Source: CAD feature listing. Evaluate the final solid. Frame: model axes, mm. Face numbers are marked on the shaded views. Give positions to 0.01 mm unless a question says otherwise; leave off trailing zeros. Order: outer loops, then holes, each group sorted by start corner. A loop starts at its lowest first (then second) coordinate and runs counter-clockwise, first axis right, second up. Notation, with made-up numbers: (68, 24) - (108, 24) arc R25 ccw to (108, 45) - close; hole circle Ø2 at (84, -21). An arc over 180 degrees is marked (long way). Write each question's results on one line, items separated by ' | '. Start each with the question number.
Item 1: Section A-A on z = -6.5. Output: boundary loops of the cut face in (x, y).
Item 2: Section B-B on y = 11.5. Output: boundary loops of the cut face in (x, z), and give its area (3 significant figures).
Item 3: Mould query, pull axis X, two halves, no side actions, for the marked faces 1, 2 and 3. Classes: released by +X, released by -X, zero draft, split by the parting line, or undercut.
Item 4: Line query: line 1 along X through (y, z) = (54.5, -15); line 2 along Z through (x, y) = (287, 40). Output: solid intervals per line, ascending.
Item 5: Contact query for a flat-ended pin moving along its axis: pin 1 Ø17.5 at (x, y) = (379.5, 26) entering from +Z. Output: stop coordinate, or through.
Item 6: Section C-C on x = 376. Output: boundary loops of the cut face in (y, z).
Autodesk Inventor part; units mm, degrees
ref_plane "YZ Plane" through (0, 0, 0) normal (1, 0, 0) x (0, 1, 0)
ref_plane "XZ Plane" through (0, 0, 0) normal (0, 1, 0) x (-1, 0, 0)
ref_plane "XY Plane" through (0, 0, 0) normal (0, 0, 1) x (1, 0, 0)
sketch "Sketch1" plane through (0, 0, 0) normal (0, 1, 0) x (-1, 0, 0)
  line L0 (0, 0) -> (-690, 0)
  line L1 (-690, 0) -> (-690, -40)
  line L2 (-690, -40) -> (0, -40)
  line L3 (0, -40) -> (0, 0)
  dimension "d0" = 690
  dimension "d1" = 40
extrude "Extrusion1" add sketch "Sketch1" along normal blind 60
sketch "Sketch3" plane through (0, 60, 0) normal (0, 1, 0) x (1, 0, 0)
  circle A0 centre (380.6828, 16.7692) radius 7.5
  line L0 (368.0221, 25.8207) -> (368.0221, 1.9407)
  line L1 (393.2421, 25.8207) -> (368.0221, 25.8207)
  line L2 (393.2421, 1.9407) -> (393.2421, 25.8207)
  line L3 (368.0221, 1.9407) -> (393.2421, 1.9407)
  line L4 (0, 0) -> (690, 0)
  line L5 (690, 40) -> (0, 40)
  line L6 (0, 40) -> (0, 0)
  line L7 (368.0221, 1.9407) -> (363.0221, 1.9407)
  line L8 (368.0221, 25.8207) -> (368.0221, 30.8207)
  line L9 (393.2421, 1.9407) -> (398.2421, 1.9407)
  line L10 (363.0221, 1.9407) -> (363.0221, 0)
  line L11 (398.2421, 1.9407) -> (398.2421, 0)
  line L12 (363.0221, 0) -> (398.2421, 0)
  line L13 (398.2421, 0) -> (398.2421, 30.8207)
  line L14 (398.2421, 30.8207) -> (363.0221, 30.8207)
  line L15 (363.0221, 30.8207) -> (363.0221, 0)
  point P0 (0, 40)
  dimension "d6" = 5
  dimension "d7" = 5
  dimension "d8" = 5
extrude "Extrusion3" cut sketch "Sketch3" against normal blind 60 contours A0 | L1 L2 L3 L0 | L8 L14 L13 L9 L2 L1 | L0 L7 L15 L14 L8 | L3 L9 L11 L4 L10 L7
sketch "Sketch4" plane through (0, 0, 0) normal (0, -1, 0) x (1, 0, 0)
  line L0 (0, 0) -> (363.0221, 0)
  line L1 (333.0221, 0) -> (268.0221, 0)
  line L2 (268.0221, 0) -> (268.0221, -25)
  line L3 (268.0221, -25) -> (333.0221, -25)
  line L4 (333.0221, -25) -> (333.0221, 0)
  line L5 (363.0221, -30.8207) -> (363.0221, 0)
  dimension "d11" = 65
  dimension "d12" = 25
  dimension "d13" = 30
extrude "Extrusion4" cut sketch "Sketch4" against normal blind 60
properties part number "Cadru_4"
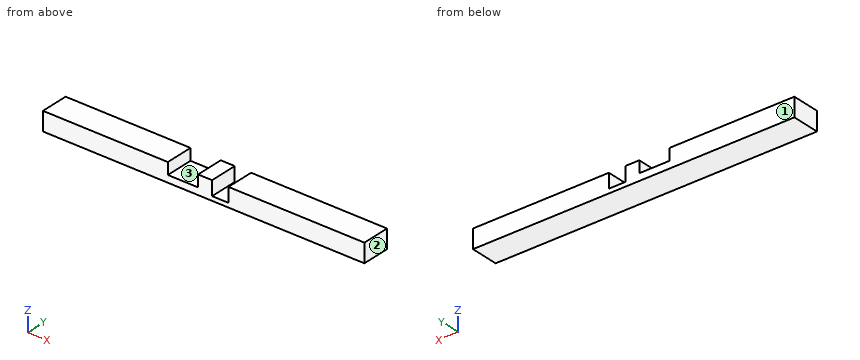
Evaluation:
1) outline: (0, 0) - (268.02, 0) - (268.02, 60) - (0, 60) - close; (333.02, 0) - (363.02, 0) - (363.02, 60) - (333.02, 60) - close; (398.24, 0) - (690, 0) - (690, 60) - (398.24, 60) - close
2) outline: (0, -40) - (690, -40) - (690, 0) - (398.24, 0) - (398.24, -30.82) - (363.02, -30.82) - (363.02, 0) - (333.02, 0) - (333.02, -25) - (268.02, -25) - (268.02, 0) - (0, 0) - close | area: 24,900 mm^2
3) face 1: zero draft | face 2: released by +X | face 3: undercut
4) line 1: x = 0 to 268.02, 333.02 to 363.02, 398.24 to 690 | line 2: z = -40 to -25
5) pin 1: stops at z = -30.82
6) outline: (0, -40) - (60, -40) - (60, -30.82) - (0, -30.82) - close
